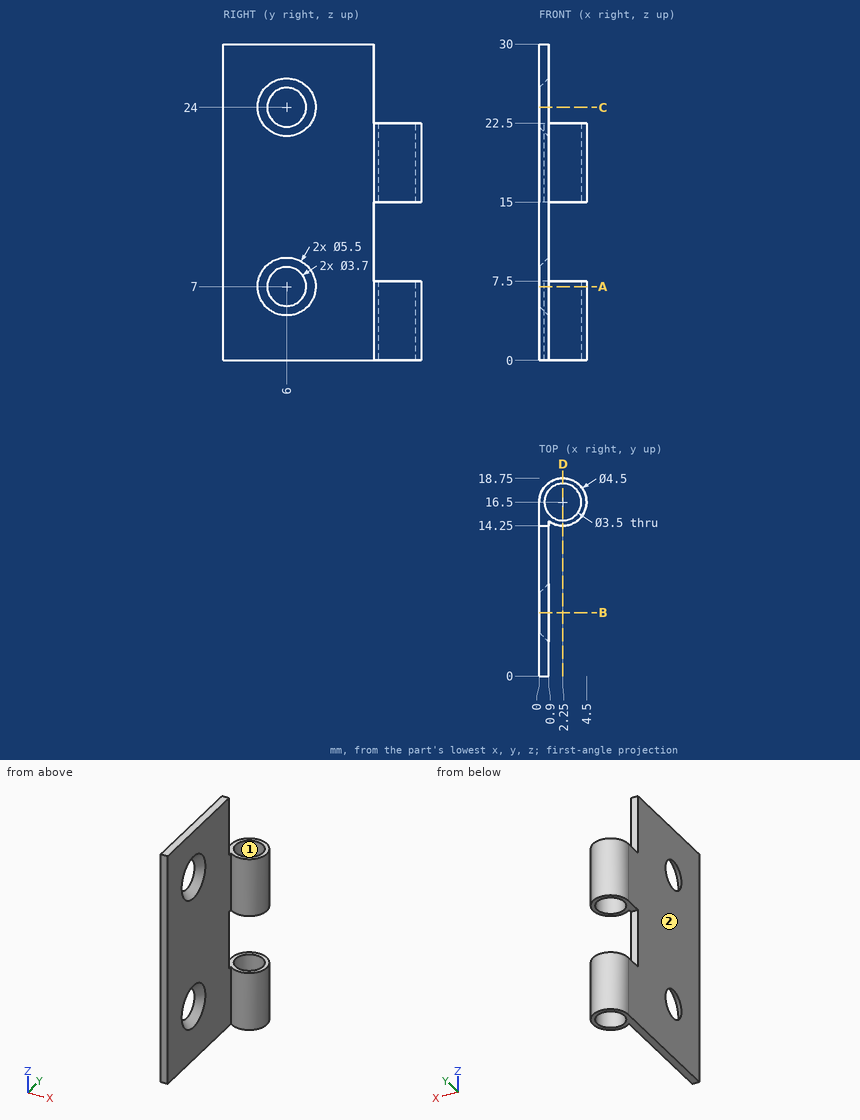
The drawing under review shows one solid part. Ordinate dimensions are in mm from its lowest x, y, z. Round coordinates to 2 decimals unless told otherwise and drop trailing zeros. Write each loop counter-clockwise with the first axis right and the second up, starting at its lowest first coordinate (ties: lowest second). Pieces come first, ordered by that corner, then holes. Notation, with made-up numbers: (-14, -15) - (0, -15) arc R20 cw to (0, -8) - close; hole circle Ø10 at (86, -18). An arc over 180 degrees is marked (long way). Put each result on its own line as item: value.
Q1. Wall thickness on probe 1 along Y at (x, z) = (2.25, 4.75); probe 2 along Z at (x, y) = (3.7, 15.25); probe 3 along X at (y, z) = (12.25, 13.75): over which ranges is each line inside the solid? List them lowest first.
Solved:
probe 1: y = 14.25 to 14.75, 18.25 to 18.75
probe 2: z = 0 to 7.5, 15 to 22.5
probe 3: x = 0 to 0.9
Q2. Insertion check: pin 1 Ø7.5 at (y, z) = (7.5, 22.5) entering from +X; pin 2 Ø10 at (y, z) = (14.5, 13.5) entering from +X; pin 3 Ø1 at (x, z) = (0.5, 27) entering from +Y. Each pin has a flat end and moves straight along its axis. Give the tip position at first contact, or say it passes through.
Solved:
pin 1: stops at x = 0.9
pin 2: stops at x = 4.5
pin 3: stops at y = 14.25
Q3. We need section C-C (z = 24). Give the boundary of the cut face in (x, y), and give its area (4 significant figures).
Solved:
outline: (0, 0) - (0.9, 0) - (0.9, 3.25) - (0, 4.15) - close; (0, 7.85) - (0.9, 8.75) - (0.9, 14.25) - (0, 14.25) - close
area: 8.685 mm2
Q4. Mouldability with a two-part tool opening along X and no side actions: class the marked faces 1 and 2 as released by +X, released by -X, zero draft, split by the parting line, or undercut.
Solved:
face 1: undercut
face 2: released by -X
Q5. We need section D-D (x = 2.25). Give the boundary of the cut face in (y, z), and give its area (3 significant figures).
Solved:
outline: (14.25, 0) - (14.75, 0) - (14.75, 7.5) - (14.25, 7.5) - close; (14.25, 15) - (14.75, 15) - (14.75, 22.5) - (14.25, 22.5) - close; (18.25, 0) - (18.75, 0) - (18.75, 7.5) - (18.25, 7.5) - close; (18.25, 15) - (18.75, 15) - (18.75, 22.5) - (18.25, 22.5) - close
area: 15.0 mm2
Q6. We need section B-B (y = 6). Give the boundary of the cut face in (x, z), and give its area (3 significant figures).
Solved:
outline: (0, 0) - (0.9, 0) - (0.9, 4.25) - (0, 5.15) - close; (0, 8.85) - (0.9, 9.75) - (0.9, 21.25) - (0, 22.15) - close; (0, 25.85) - (0.9, 26.75) - (0.9, 30) - (0, 30) - close
area: 18.7 mm2
Q7. We need section A-A (z = 7). Give the boundary of the cut face in (x, y).
Solved:
outline: (0, 0) - (0.9, 0) - (0.9, 3.25) - (0, 4.15) - close; (0, 7.85) - (0.9, 8.75) - (0.9, 14.7) arc R2.25 ccw (long way) to (0, 16.5) - close; hole circle Ø3.5 at (2.25, 16.5)
